Could you check a few things on this model? Use its own coordinates, in mm. Round coordinates to 2 decimals unless told otherwise and drop trailing zeros. Order: outer loops, then holes, each group sorted by start corner. A loop starts at its lowest first (then second) coordinate and runs counter-clockwise, first axis right, second up. Notation, with made-up numbers: (67, 86.5) - (74, 86.5) arc R18 ccw to (74, 120.5) - close; hole circle Ø6 at (-14, 68.5). An arc over 180 degrees is marked (long way). Return JSON: item names as keys, results as strings. Group by question number.
from build123d import *

# Parameters (mm, degrees)
MODEL_R             = 2
MODEL_R_2           = 2.45
MODEL_W             = 352.775
MODEL_H             = 95.6
BOSS_EXTRUDE1_DEPTH = 3


with BuildPart() as part:
    # Model → Boss-Extrude1 (new body)
    with BuildSketch(Plane.XY):
        with BuildLine():
            Line((0, 108.6), (0, 5))
            ThreePointArc((0, 5), (1.464466094, 1.464466094), (5, 0))
            Line((5, 0), (365.775, 0))
            ThreePointArc((365.775, 0), (369.310533906, 1.464466094), (370.775, 5))
            Line((370.775, 5), (370.775, 108.6))
            ThreePointArc((370.775, 108.6), (369.310533906, 112.135533906), (365.775, 113.6))
            Line((365.775, 113.6), (5, 113.6))
            ThreePointArc((5, 113.6), (1.464466094, 112.135533906), (0, 108.6))
        make_face()
        with Locations((85.3875, 107.6)):
            Circle(MODEL_R, mode=Mode.SUBTRACT)
        with Locations((285.3875, 107.6)):
            Circle(MODEL_R, mode=Mode.SUBTRACT)
        with Locations((85.3875, 6)):
            Circle(MODEL_R, mode=Mode.SUBTRACT)
        with Locations((185.3875, 6)):
            Circle(MODEL_R, mode=Mode.SUBTRACT)
        with Locations((285.3875, 6)):
            Circle(MODEL_R, mode=Mode.SUBTRACT)
        with Locations((175.3875, 109.1)):
            Circle(MODEL_R_2, mode=Mode.SUBTRACT)
        with Locations((195.3875, 109.1)):
            Circle(MODEL_R_2, mode=Mode.SUBTRACT)
        with Locations((185.3875, 56.8)):
            Rectangle(MODEL_W, MODEL_H, mode=Mode.SUBTRACT)
        Polygon((365.947431604, 110.609548911), (367.784548911, 108.772431604), (367.112117307, 106.262882693), (364.602568396, 105.590451089), (362.765451089, 107.427568396), (363.437882693, 109.937117307), align=None, mode=Mode.SUBTRACT)
        Polygon((4.827568396, 110.609548911), (2.990451089, 108.772431604), (3.662882693, 106.262882693), (6.172431604, 105.590451089), (8.009548911, 107.427568396), (7.337117307, 109.937117307), align=None, mode=Mode.SUBTRACT)
        Polygon((365.947431604, 2.990451089), (367.784548911, 4.827568396), (367.112117307, 7.337117307), (364.602568396, 8.009548911), (362.765451089, 6.172431604), (363.437882693, 3.662882693), align=None, mode=Mode.SUBTRACT)
        Polygon((4.827568396, 2.990451089), (2.990451089, 4.827568396), (3.662882693, 7.337117307), (6.172431604, 8.009548911), (8.009548911, 6.172431604), (7.337117307, 3.662882693), align=None, mode=Mode.SUBTRACT)
        Polygon((126.799038106, 2.25), (124.200961894, 2.25), (122.901923789, 4.5), (124.200961894, 6.75), (126.799038106, 6.75), (128.098076211, 4.5), align=None, mode=Mode.SUBTRACT)
        Polygon((126.799038106, 111.35), (124.200961894, 111.35), (122.901923789, 109.1), (124.200961894, 106.85), (126.799038106, 106.85), (128.098076211, 109.1), align=None, mode=Mode.SUBTRACT)
        Polygon((243.975961894, 2.25), (246.574038106, 2.25), (247.873076211, 4.5), (246.574038106, 6.75), (243.975961894, 6.75), (242.676923789, 4.5), align=None, mode=Mode.SUBTRACT)
        Polygon((243.975961894, 111.35), (246.574038106, 111.35), (247.873076211, 109.1), (246.574038106, 106.85), (243.975961894, 106.85), (242.676923789, 109.1), align=None, mode=Mode.SUBTRACT)
    extrude(amount=BOSS_EXTRUDE1_DEPTH)


solid = part.part
1) Will this pin go through, and if not, where does the flat tip stop? pin 1 (4.5 mm diameter, centred on x = 195.39, y = 109.1, fed in from +Z).
2) I want a section at A-A, the plane y = 13. List the corners of the cut face in (x, z) for me (3 decimals).
3) I want a section at C-C, the plane z = 0.8. Give the number of separate pieces and of enclosed holes in the cut face, plus the area to 3 significant figures.
4) If I drill on line 1 along Y through (x, z) = (180, 1.3); line 2 along X through (y, z) = (40, 0.85) (3 decimals), over which ranges is the centre line in solid material (lowest first)? Write a range as from..to.
5) I want a section at B-B, the plane x = 226.5. List the corners of the cut face in (y, z) for me, plus the area to 3 significant figures.
Outcome:
{
 "1": {"pin 1": "through"},
 "2": {"outline": "(0, 0) - (9, 0) - (9, 3) - (0, 3) - close; (361.775, 0) - (370.775, 0) - (370.775, 3) - (361.775, 3) - close"},
 "3": {"separate pieces": "1", "enclosed holes": "16", "area": "8,130 mm^2"},
 "4": {"line 1": "0..9, 104.6..113.6", "line 2": "0..9, 361.775..370.775"},
 "5": {"outline": "(0, 0) - (9, 0) - (9, 3) - (0, 3) - close; (104.6, 0) - (113.6, 0) - (113.6, 3) - (104.6, 3) - close", "area": "54.0 mm^2"}
}
